Could you check a few things on this model? Use its own coordinates, in mm. A direction names the side the tool comes from. Round coordinates to 2 decimals unless told otherwise and drop trailing zeros. Loops run counter-clockwise (first coordinate to the right, second up) from the corner with the lowest first, then second, coordinate; pieces in that order, holes last. Notation, with made-up numbers: M 51.25,14 L 92.25,14 A25 ccw 92.25,28 Z; hole C 15,36.25 d10. An arc over 180 degrees is marked long. One line per item, written item: value. Start each with the question number.
Q1. Imagine slicing it at C-C (z = 8). Please give me the cut outline in (x, y) (3 decimals), then the cut area to 3 significant figures.
Q2. Which directions (+Z, -Z, +X, -X, +Y, -Y) give clear straight access to the entire face, cutting with the end or side of a thin tool? Please do faces 1 (the face through (0, 9, 0)), 2 (the face through (-4.86, 19.575, 6.719)).
Q3. Thinking about a two-plate mould opening in X: for faces 3 (the face through (-6, 14, 9)), 4 (the face through (-6, 14, 11)), 5 (the face through (5.91, -8.43, 2.96)), which applies, released by +X, released by -X, zero draft, split by the parting line, or undercut?
Q4. Imagine slicing it at B-B (y = 13.75). Please give me the cut outline in (x, z) (3 decimals).
Q5. I'm going to push flat-ended pins straight in: pin 1 Ø7 at (x, y) = (-5.625, 13.75) entering from -Z; pin 2 Ø2 at (y, z) = (-2, 3.5) entering from +X; pin 3 Ø4 at (y, z) = (5, 6) entering from +X. Where does each tip first touch, or does it pass through?
Q6. Imagine slicing it at A-A (z = 1.5). Please give me the cut outline in (x, y) (3 decimals), then the cut area to 3 significant figures.
Q7. Please list where these lines run through material, in increasing order: line 1 along Y through (x, z) = (-5.5, 8.75); line 2 along Z through (x, y) = (-1, 15.5); line 3 along Y through (x, z) = (-4, 6).
from build123d import *

# Parameters (mm, degrees)
CROQUIS1_R              = 25
SALIENTE_EXTRUIR1_DEPTH = 11
REDONDEO1_R             = 5
CROQUIS2_R              = 5.875
CORTAR_EXTRUIR1_DEPTH   = 9
CROQUIS3_R              = 7
CORTAR_EXTRUIR2_DEPTH   = 4.5


with BuildPart() as part:
    # Croquis1 → Saliente-Extruir1 (new body)
    with BuildSketch(Plane.XY):
        with Locations((-5.625, 13.75)):
            Circle(CROQUIS1_R)
    extrude(amount=SALIENTE_EXTRUIR1_DEPTH)

    # Redondeo1
    redondeo1_edges = [part.edges().sort_by_distance(p)[0] for p in [
        (-30.625, 13.75, 11),
    ]]
    fillet(redondeo1_edges, radius=REDONDEO1_R)

    # Croquis2 → Cortar-Extruir1 (cut)
    with BuildSketch(Plane(origin=(0, 0, 0), x_dir=(-1, 0, 0), z_dir=(0, 0, -1))):
        with Locations((5.625, 13.75)):
            Circle(CROQUIS2_R)
    extrude(amount=-CORTAR_EXTRUIR1_DEPTH, mode=Mode.SUBTRACT)

    # Croquis3 → Cortar-Extruir2 (cut)
    with BuildSketch(Plane(origin=(0, 0, 0), x_dir=(-1, 0, 0), z_dir=(0, 0, -1))):
        with Locations((5.625, 13.75)):
            Circle(CROQUIS3_R)
    extrude(amount=-CORTAR_EXTRUIR2_DEPTH, mode=Mode.SUBTRACT)


solid = part.part
Report:
1. outline: C -5.625,13.75 d49.165; hole C -5.625,13.75 d11.75
1. area: 1,790 mm²
2. face 1: -Z, +X, -X, +Y, -Y
2. face 2: -Z
3. face 3: undercut
3. face 4: zero draft
3. face 5: split by the parting line
4. outline: M -30.625,0 L -12.625,0 L -12.625,4.5 L -11.5,4.5 L -11.5,9 L 0.25,9 L 0.25,4.5 L 1.375,4.5 L 1.375,0 L 19.375,0 L 19.375,6 A5 ccw 14.375,11 L -25.625,11 A5 ccw -30.625,6 Z
5. pin 1: stops at z = 9
5. pin 2: stops at x = 14.56
5. pin 3: stops at x = 18.45
6. outline: C -5.625,13.75 d50; hole C -5.625,13.75 d14
6. area: 1,810 mm²
7. line 1: y = -10.43 to 7.88, 19.62 to 37.93
7. line 2: z = 9 to 11
7. line 3: y = -11.2 to 8.1, 19.4 to 38.7
